```python
from build123d import *

# Parameters (mm, degrees)
F1_DEPTH = 2526
F2_R     = 100


with BuildPart() as f1:
    # F0 (on Front) → F1 (new body)
    with BuildSketch(Plane.XZ):
        with BuildLine():
            ThreePointArc((-685, 200), (-677.4536303253, 691.6975376497), (-654.8216297668, 1182.9319102019))
            Line((-654.8216297668, 1182.9319102019), (-657.8159792684, 1183.1159511275))
            ThreePointArc((-657.8159792684, 1183.1159511275), (-680.4522173679, 691.7896014733), (-688, 200))
            Line((-688, 200), (-685, 200))
        make_face()
    extrude(amount=F1_DEPTH)

    # F2
    f2_edges = [f1.edges().sort_by_distance(p)[0] for p in [
        (-686.5, -2526, 200),
        (-686.5, 0, 200),
    ]]
    fillet(f2_edges, radius=F2_R)


solid = f1.part
```
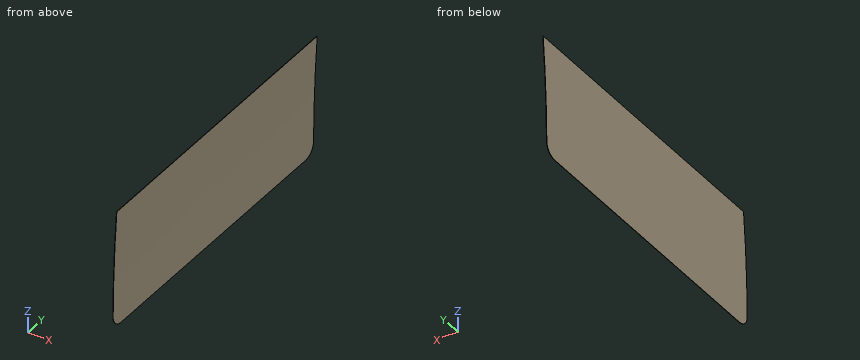
The listing builds one solid part. Answer for the finished solid, in the listing's coordinates (mm). Give positions to 0.01 mm unless a question says otherwise; leave off trailing zeros. Order: outer loops, then holes, each group sorted by start corner. A loop starts at its lowest first (then second) coordinate and runs counter-clockwise, first axis right, second up. Notation, with made-up numbers: (-28, 84) -> (6, 84) arc R25 cw to (6, 104) -> close; hole circle Ø1 at (17, 75). An arc over 180 degrees is marked (long way). Answer as a JSON object with one key per item and string values. Group by question number.
Item 1: Consider L1, parallel to X at y = -1040.5, z = 245.5; L2, parallel to X at y = -2049.5, z = 294.5. Determine where each line is inside the solid, lowest interval first. Write a range as from..to.
Item 2: The part is cut by section B-B on z = 951.5. Write down the section's boundary in (x, y), and give its area (3 significant figures).
Item 3: The part is cut by section A-A on y = -2088.5. Write down the section's boundary in (x, z).
Result set:
{
 "1": {"L1": "-687.94..-684.94", "L2": "-687.72..-684.72"},
 "2": {"outline": "(-670.37, -2526) -> (-667.37, -2526) -> (-667.37, 0) -> (-670.37, 0) -> close", "area": "7,590 mm²"},
 "3": {"outline": "(-688, 200) -> (-685, 200) arc R16022.5 cw to (-654.82, 1182.93) -> (-657.82, 1183.12) arc R16025.5 ccw to start"}
}
